```python
from build123d import *

# Parameters (mm, degrees)
F0_R      = 30.25
F0_R_2    = 25.25
F1_DEPTH  = 18
F2_R      = 35.25
F2_R_2    = 30.25
F2_R_3    = 25.25
F3_DEPTH  = 7
F4_R      = 30.25
F4_R_2    = 25.25
F5_DEPTH  = 10
F6_R      = 35.25
F6_R_2    = 30.25
F6_R_3    = 25.25
F7_DEPTH  = 7
F8_R      = 2
F10_DEPTH = 50
F11_R     = 2
F13_DEPTH = 50
F14_R     = 2
F15_SIZE2 = 4.99999
F15_SIZE  = 4.99999


# Not quite as in the source:
# - a fillet or chamfer is up to 0.001 mm smaller than in the source, because OpenCascade refuses the exact size


with BuildPart() as f1:
    # F0 (on Top) → F1 (new body)
    with BuildSketch(Plane.XY):
        Circle(F0_R)
        Circle(F0_R_2, mode=Mode.SUBTRACT)
    extrude(amount=F1_DEPTH)

    # F2 (on face) → F3 (join)
    with BuildSketch(Plane.XY.offset(18)):
        Circle(F2_R)
        Circle(F2_R_2, mode=Mode.SUBTRACT)
        Circle(F2_R_2)
        Circle(F2_R_3, mode=Mode.SUBTRACT)
    extrude(amount=F3_DEPTH)

    # F4 (on face) → F5 (join)
    with BuildSketch(Plane.XY.offset(25)):
        Circle(F4_R)
        Circle(F4_R_2, mode=Mode.SUBTRACT)
    extrude(amount=F5_DEPTH)

    # F6 (on face) → F7 (join)
    with BuildSketch(Plane.XY.offset(35)):
        Circle(F6_R)
        Circle(F6_R_2, mode=Mode.SUBTRACT)
        Circle(F6_R_2)
        Circle(F6_R_3, mode=Mode.SUBTRACT)
    extrude(amount=F7_DEPTH)

    # F8
    f8_edges = [f1.edges().sort_by_distance(p)[0] for p in [
        (-25.25, 0, 42),
    ]]
    fillet(f8_edges, radius=F8_R)

    # F9 (on Front) → F10 (cut)
    with BuildSketch(Plane.XZ):
        Polygon((-6, 0), (0, 0), (0, 8.0120034479), (3.5, 8.0120034479), (3.5, 4), (9.5, 4), (9.5, 13), (-6, 13), align=None)
    extrude(amount=-F10_DEPTH, mode=Mode.SUBTRACT)

    # F11
    f11_edges = [f1.edges().sort_by_distance(p)[0] for p in [
        (9.5, 26.05713, 13),
        (-6, 27.08788, 13),
        (3.5, 27.526544, 4),
        (9.5, 26.05713, 4),
    ]]
    fillet(f11_edges, radius=F11_R)

    # F12 (on Front) → F13 (cut)
    with BuildSketch(Plane.XZ):
        Polygon((-0.0314122736, -0.0527559742), (5.9685877264, -0.0527559742), (5.9685877264, 12.9472440258), (-9.5314122736, 12.9472440258), (-9.5314122736, 3.9472440258), (-3.5314122736, 3.9472440258), (-3.5314122736, 7.9592474737), (-0.0314122736, 7.9592474737), align=None)
    extrude(amount=F13_DEPTH, mode=Mode.SUBTRACT)

    # F14
    f14_edges = [f1.edges().sort_by_distance(p)[0] for p in [
        (-9.531412, -26.045535, 12.947244),
        (-9.531412, -26.045535, 3.947244),
        (-3.531412, -27.522498, 3.947244),
        (5.968588, -27.094881, 12.947244),
    ]]
    fillet(f14_edges, radius=F14_R)

    # F15 (size 5 and 5 in the source; OpenCascade refuses exactly that, so slightly less here)
    f15_edges = [f1.edges().sort_by_distance(p)[0] for p in [
        (-35.25, 0, 18),
        (-35.25, 0, 42),
    ]]
    chamfer(f15_edges, length=F15_SIZE, length2=F15_SIZE2)


solid = f1.part
```
The model under review builds one solid part; all positions refer to its coordinate system, in mm. A direction names the side the tool comes from. Round coordinates to 2 decimals unless told otherwise and drop trailing zeros. Write each loop counter-clockwise with the first axis right and the second up, starting at its lowest first coordinate (ties: lowest second). Pieces come first, ordered by that corner, then holes. Notation, with made-up numbers: (54.5, 58.5) - (73.5, 58.5) arc R22 ccw to (73.5, 74.5) - close; hole circle Ø6 at (-24, -36). An arc over 180 degrees is marked (long way). Use one line per item in the form item = value.
Q1. Draft analysis for pull direction X (two halves, no side actions). For faces 1 (the conical face through (-6.625, -29.836, 18.313)), 2 (the flat face through (25, 5, 0)), 3 (the flat face through (-6, 27, 6)), state which applies: +X half, -X half, draft (parallel to the pull), parting line (faces both ways), or undercut.
Answer key:
face_1 = parting line
face_2 = draft
face_3 = undercut
Q2. Consider section A-A (z = 16). State the section outline as (x, y) points, and give its area (3 significant figures).
Answer key:
outline = circle Ø60.5 at (0, 0); hole circle Ø50.5 at (0, 0)
area = 872 mm2
Q3. Consider section B-B (x = 8.5). State how many separate pieces and enclosed holes the cut face has, and give its area (3 significant figures).
Answer key:
separate_pieces = 3
enclosed_holes = 0
area = 488 mm2
Q4. Consider section C-C (z = 24). State the section outline as (x, y) points.
Answer key:
outline = circle Ø70.5 at (0, 0); hole circle Ø50.5 at (0, 0)
Q5. Tool access review of faces 4 (the cylindrical face through (13.959, -26.837, 8.874)), 5 (the flat face through (2, 28, 8.012)), 6 (the flat face through (-9.531, -26, 8)), 7 (the flat face through (2, 28, 13)): name each direction out of +Z, -Z, +X, -X, +Y, -Y from which nothing blocks a thin tool from reaching the whole face with its end or side.
Answer key:
face_4 = -Z
face_5 = +Y, -Y
face_6 = -Y
face_7 = +Y
Q6. For line 1 (Y direction, x = 7.5, z = 33.5); line 2 (Y direction, x = 0, z = 16), list the stretches that pass through material, from the lowest coordinate up. Write a range as [from, to].
Answer key:
line_1 = [-29.31, -24.11], [24.11, 29.31]
line_2 = [-30.25, -25.25], [25.25, 30.25]
Q7. Insertion check: pin 1 Ø1 at (x, z) = (8.5, 29) entering from +Y; pin 2 Ø5.5 at (y, z) = (-28, 2.5) entering from +X; pin 3 Ø6 at (x, y) = (23, -7) entering from -Z; pin 4 Ø3 at (x, z) = (9, 22.5) entering from -Y. Each pin has a flat end and moves straight along its axis. Give the tip position at first contact, or say it passes through.
Answer key:
pin_1 = 29.17
pin_2 = 16.66
pin_3 = 0
pin_4 = -34.42
